```python
from build123d import *

# Parameters (mm, degrees)
F0_W      = 16
F0_H      = 34
F1_DEPTH  = 16
F2_W      = 10
F2_H      = 10
F3_DEPTH  = 30
F4_W      = 10
F4_H      = 10
F5_DEPTH  = 30
F6_R      = 1.5
F7_DEPTH  = 16
F8_W      = 16
F8_H      = 16
F9_DEPTH  = 34
F10_W     = 10
F10_H     = 10
F11_DEPTH = 30
F12_R     = 1.5
F13_DEPTH = 16


with BuildPart() as f1:
    # F0 (on Top) → F1 (new body)
    with BuildSketch(Plane.XY):
        Polygon((25, 16), (-25, 16), (-25, 0), (-9, 0), (25, 0), align=None)
        with Locations((-17, -17)):
            Rectangle(F0_W, F0_H)
    extrude(amount=F1_DEPTH)

    # F2 (on face) → F3 (cut)
    with BuildSketch(Plane.YZ.offset(25)):
        with Locations((8, 8)):
            Rectangle(F2_W, F2_H)
    extrude(amount=-F3_DEPTH, mode=Mode.SUBTRACT)

    # F4 (on face) → F5 (cut)
    with BuildSketch(Plane.XZ.offset(34)):
        with Locations((-17, 8)):
            Rectangle(F4_W, F4_H)
    extrude(amount=-F5_DEPTH, mode=Mode.SUBTRACT)

    # F6 (on face) → F7 (cut)
    with BuildSketch(Plane.XY.offset(16)):
        with Locations((-17, -26)):
            Circle(F6_R)
        with Locations((17, 8)):
            Circle(F6_R)
    extrude(amount=-F7_DEPTH, mode=Mode.SUBTRACT)

    # F8 (on face) → F9 (join)
    with BuildSketch(Plane.XY.offset(16)):
        with Locations((-17, 8)):
            Rectangle(F8_W, F8_H)
    extrude(amount=F9_DEPTH)

    # F10 (on face) → F11 (cut)
    with BuildSketch(Plane.XY.offset(50)):
        with Locations((-17, 8)):
            Rectangle(F10_W, F10_H)
    extrude(amount=-F11_DEPTH, mode=Mode.SUBTRACT)

    # F12 (on face) → F13 (cut)
    with BuildSketch(Plane.XZ):
        with Locations((-17, 42)):
            Circle(F12_R)
    extrude(amount=-F13_DEPTH, mode=Mode.SUBTRACT)


solid = f1.part
```
Check sheet for the modelled part. Datum: model origin and axes. Units: mm. A direction names the side the tool comes from. Give positions to 0.01 mm unless a question says otherwise; leave off trailing zeros. Loops run counter-clockwise (first coordinate to the right, second up) from the corner with the lowest first, then second, coordinate; pieces in that order, holes last. Notation, with made-up numbers: (7, -35) - (52, -35) arc R22 ccw to (52, -9) - close; hole circle Ø4 at (-36, 59.25). An arc over 180 degrees is marked (long way). One line per question, with ' | ' between items. Start each with the question number.
1. Draft check along Y on faces 4 (the cylindrical face through (-17.325, 1.479, 40.536)), 5 (the flat face through (-5, 8, 8)), 6 (the flat face through (10, 3, 8)), 7 (the flat face through (8, 0, 8)). Enter one of: released by +Y, released by -Y, zero draft, split by the parting line, or undercut.
2. Cross-section at A-A, the plane y = 8. Enter the section's corners in (x, z), plus the area to 3 significant figures.
3. Material ranges on line 1 along X through (y, z) = (-23, 4.5); line 2 along Y through (x, z) = (-17, 14.8); line 3 along Z through (x, y) = (-4, 12), recorded low to high. Write a range as [from, to].
4. Cross-section at D-D, the plane x = 17. Enter the section's corners in (y, z), plus the area to 3 significant figures.
5. Gauge pin test, flat ends, axial feed: pin 1 Ø8 at (x, z) = (-17, 27.5) entering from -Y; pin 2 Ø12 at (y, z) = (-22, 22.5) entering from -X; pin 3 Ø11 at (x, y) = (6.5, 7.5) entering from +Z; pin 4 Ø2 at (y, z) = (-0.5, 32) entering from +X. Record the tip position at first contact, or that the pin passes through.
6. Cross-section at B-B, the plane z = 27.5. Enter the section's corners in (x, y).
7. Set-up check for faces 1 (the flat face through (-17, 8, 20)), 2 (the flat face through (10, 13, 8)), 3 (the flat face through (-17, -4, 8)): record each of +Z, -Z, +X, -X, +Y, -Y from which the full face is reachable in a straight line by a thin tool's end or side.
8. Cross-section at C-C, the plane z = 42. Enter the section's corners in (x, y).
Check result:
1) face 4: zero draft | face 5: undercut | face 6: undercut | face 7: released by -Y
2) outline: (-25, 0) - (15.5, 0) - (15.5, 3) - (-5, 3) - (-5, 13) - (15.5, 13) - (15.5, 16) - (-9, 16) - (-9, 50) - (-12, 50) - (-12, 20) - (-22, 20) - (-22, 50) - (-25, 50) - close; (18.5, 0) - (25, 0) - (25, 3) - (18.5, 3) - close; (18.5, 13) - (25, 13) - (25, 16) - (18.5, 16) - close | area: 726 mm2
3) line 1: x = [-25, -22], [-12, -9] | line 2: y = [-34, -27.5], [-24.5, 16] | line 3: z = [0, 3], [13, 16]
4) outline: (0, 0) - (6.5, 0) - (6.5, 3) - (3, 3) - (3, 13) - (6.5, 13) - (6.5, 16) - (0, 16) - close; (9.5, 0) - (16, 0) - (16, 16) - (9.5, 16) - (9.5, 13) - (13, 13) - (13, 3) - (9.5, 3) - close | area: 138 mm2
5) pin 1: stops at y = 0 | pin 2: passes through | pin 3: stops at z = 16 | pin 4: stops at x = -9
6) outline: (-25, 0) - (-9, 0) - (-9, 16) - (-25, 16) - close; hole (-22, 3) - (-12, 3) - (-12, 13) - (-22, 13) - close
7) face 1: +Z | face 2: +X | face 3: -Y
8) outline: (-25, 0) - (-18.5, 0) - (-18.5, 3) - (-22, 3) - (-22, 13) - (-18.5, 13) - (-18.5, 16) - (-25, 16) - close; (-15.5, 0) - (-9, 0) - (-9, 16) - (-15.5, 16) - (-15.5, 13) - (-12, 13) - (-12, 3) - (-15.5, 3) - close
